Work out the finished part from the listing and answer in its coordinate system (mm). Face numbers are marked on the shaded views. A direction names the side the tool comes from. Give positions to 0.01 mm unless a question says otherwise; leave off trailing zeros. Write each loop counter-clockwise with the first axis right and the second up, starting at its lowest first coordinate (ties: lowest second). Pieces come first, ordered by that corner, then holes. Notation, with made-up numbers: (-8, 86.25) -> (-2, 86.25) arc R31 cw to (-2, 124.25) -> close; hole circle Ø9 at (-18.75, 68.5). An arc over 180 degrees is marked (long way). Use a Markdown table: item, result. Add a question column.
Q1. Section B-B, the plane z = -6.5 is taken. Give the vertices of the cut face in (x, y).
Q2. Consider line 1 (Z direction, x = -4, y = -2.5); line 2 (Z direction, x = 2.5, y = 3.25); line 3 (Z direction, x = -14, y = 1.75). Determine where each line is inside the solid, lowest interval first.
Q3. Section D-D, the plane y = -1.75 is taken. Give the vertices of the cut face in (x, z) (3 decimals).
Q4. Section A-A, the plane x = 8 is taken. Give the vertices of the cut face in (y, z).
Q5. For a pull along X with two mould halves and no side action, classify the marked faces 4, 5, 6 and 7 as pulls with the +X half, pulls with the -X half, needs draft (parallel to the pull), parting line crosses it, or undercut.
Q6. Each of these flat-tipped pins is pushed along its axis until it touches: pin 1 Ø2.5 at (y, z) = (0, 2) entering from -X; pin 2 Ø4 at (x, y) = (-14, -0.5) entering from -Z; pin 3 Ø1.2 at (y, z) = (0, 15.5) entering from +X (3 decimals); pin 4 Ø1 at (x, z) = (-12, -2) entering from -Y. Where does it stop, or does it pass through?
Q7. Section C-C, the plane x = -6 is taken. Give the vertices of the cut face in (y, z).
Q8. For the marked faces 1, 2 and 3, determine the directions among +Z, -Z, +X, -X, +Y, -Y from which every point of the face is accessible in a straight line to the end or side of a thin tool.
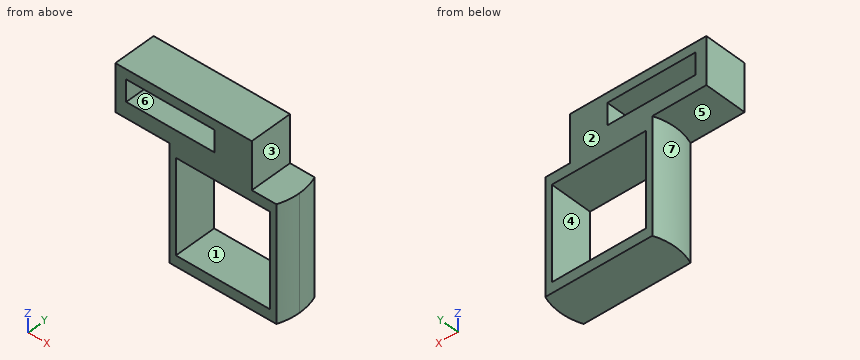
from build123d import *

# Parameters (mm, degrees)
F0_W          = 16.5766410064
F0_H          = 4.0903398767
F1_DEPTH      = 4
F1_DEPTH_BACK = 4
F3_DEPTH      = 21.7


with BuildPart() as f1:
    # F0 (on Front) → F1 (new body, two sides)
    with BuildSketch(Plane.XZ) as f1_sk:
        Polygon((-10.85, 10.85), (-10.85, 0), (-10.85, -10.85), (0, -10.85), (10.85, -10.85), (10.85, 0), (10.85, 10.85), (5.425, 10.85), (0, 10.85), align=None)
        Polygon((8.85, 8.85), (8.85, 0), (8.85, -8.85), (0, -8.85), (-8.85, -8.85), (-8.85, 0), (-8.85, 8.85), (0, 8.85), align=None, mode=Mode.SUBTRACT)
        Polygon((-20.2364195138, 10.85), (-10.85, 10.85), (0, 10.85), (5.425, 10.85), (5.425, 19.7520367801), (-20.2364195138, 19.7520367801), align=None)
        with Locations((-9.9029276753, 15.8769781701)):
            Rectangle(F0_W, F0_H, mode=Mode.SUBTRACT)
    extrude(amount=F1_DEPTH)
    extrude(f1_sk.sketch, amount=-F1_DEPTH_BACK)

    # F2 (on face) → F3 (cut)
    with BuildSketch(Plane(origin=(0, 0, -10.85), x_dir=(1, 0, 0), z_dir=(0, 0, -1))):
        with BuildLine():
            Line((13.9217844345, 4.8126999282), (9.694906495, 4.8126999282))
            ThreePointArc((9.694906495, 4.8126999282), (9.8845588749, 4.4100780486), (10.0574993187, 4))
            Line((10.0574993187, 4), (10.85, 4))
            Line((10.85, 4), (10.85, -4))
            Line((10.85, -4), (10.0574993187, -4))
            ThreePointArc((10.0574993187, -4), (9.8311449192, -4.52790041), (9.5771050518, -5.0430498086))
            Line((9.5771050518, -5.0430498086), (13.9217844345, -5.0430498086))
            Line((13.9217844345, -5.0430498086), (13.9217844345, 4.8126999282))
        make_face()
        with BuildLine():
            Line((10.85, 4), (10.0574993187, 4))
            ThreePointArc((10.0574993187, 4), (10.6304521223, 2.0363644618), (10.8237374574, 0))
            ThreePointArc((10.8237374574, 0), (10.6304521223, -2.0363644618), (10.0574993187, -4))
            Line((10.0574993187, -4), (10.85, -4))
            Line((10.85, -4), (10.85, 4))
        make_face()
        with BuildLine():
            ThreePointArc((-10.0574993187, -4), (-10.8237374574, 0), (-10.0574993187, 4))
            Line((-10.0574993187, 4), (-10.85, 4))
            Line((-10.85, 4), (-10.85, -4))
            Line((-10.85, -4), (-10.0574993187, -4))
        make_face()
    extrude(amount=-F3_DEPTH, mode=Mode.SUBTRACT)


solid = f1.part
Result set:
| question | item | result |
|---|---|---|
| 1 | outline | (-10.06, -4) -> (-8.85, -4) -> (-8.85, 4) -> (-10.06, 4) arc R10.82 ccw to start; (8.85, -4) -> (10.06, -4) arc R10.82 ccw to (10.06, 4) -> (8.85, 4) -> close |
| 2 | line 1 | z = -10.85 to -8.85, 8.85 to 13.83, 17.92 to 19.75 |
| 2 | line 2 | z = -10.85 to -8.85, 8.85 to 19.75 |
| 2 | line 3 | z = 10.85 to 13.83, 17.92 to 19.75 |
| 3 | outline | (-20.236, 10.85) -> (-10.681, 10.85) -> (-10.681, -10.85) -> (10.681, -10.85) -> (10.681, 10.85) -> (5.425, 10.85) -> (5.425, 19.752) -> (-20.236, 19.752) -> close; hole (-18.191, 13.832) -> (-1.615, 13.832) -> (-1.615, 17.922) -> (-18.191, 17.922) -> close; hole (-8.85, -8.85) -> (8.85, -8.85) -> (8.85, 8.85) -> (-8.85, 8.85) -> close |
| 4 | outline | (-4, -10.85) -> (4, -10.85) -> (4, -8.85) -> (-4, -8.85) -> close; (-4, 8.85) -> (4, 8.85) -> (4, 10.85) -> (-4, 10.85) -> close |
| 5 | face 4 | undercut |
| 5 | face 5 | needs draft |
| 5 | face 6 | undercut |
| 5 | face 7 | pulls with the -X half |
| 6 | pin 1 | stops at x = -10.82 |
| 6 | pin 2 | stops at z = 10.85 |
| 6 | pin 3 | stops at x = 5.425 |
| 6 | pin 4 | passes through |
| 7 | outline | (-4, -10.85) -> (4, -10.85) -> (4, -8.85) -> (-4, -8.85) -> close; (-4, 8.85) -> (4, 8.85) -> (4, 13.83) -> (-4, 13.83) -> close; (-4, 17.92) -> (4, 17.92) -> (4, 19.75) -> (-4, 19.75) -> close |
| 8 | face 1 | +Y, -Y |
| 8 | face 2 | +Z, -Z, +X, -X, +Y |
| 8 | face 3 | +Z, +X, +Y, -Y |
